Work out the finished part from the listing and answer in its coordinate system (mm). Face numbers are marked on the shaded views. A direction names the side the tool comes from. Round coordinates to 2 decimals unless told otherwise and drop trailing zeros. Order: outer loops, then holes, each group sorted by start corner. A loop starts at its lowest first (then second) coordinate and runs counter-clockwise, first axis right, second up. Notation, with made-up numbers: (-30.5, 29) -> (10.5, 29) arc R11 cw to (10.5, 39) -> close; hole circle Ø3 at (43, -16.75). An arc over 180 degrees is marked (long way). Use a Markdown table: item, result. Add a question column.
Item 1: A cutting plane is placed at C-C, the plane x = 17. Determine the outline of the cut face in (y, z), plus the area to 3 significant figures.
Item 2: A cutting plane is placed at D-D, the plane z = 23.5. Determine the outline of the cut face in (x, y).
Item 3: Find the intervals of material crossed by L1, parallel to Y at x = 62, z = 6.5; L2, parallel to X at y = 72.5, z = 1.5; L3, parallel to Y at x = 41.5, z = 6.75, in increasing order. Write a range as [from, to].
Item 4: For a pull along Y with two mould halves and no side action, classify the marked faces 6, 7, 8 and 9 as +Y half, -Y half, draft (parallel to the pull), parting line (faces both ways), or undercut.
Item 5: A cutting plane is placed at B-B, the plane y = 71. Determine the outline of the cut face in (x, z), plus the area to 3 significant figures.
Item 6: A cutting plane is placed at A-A, the plane z = 9.5. Determine the outline of the cut face in (x, y).
Item 7: A tool of negligible diameter and unlimited length cuts with its end or side. For the marked faces 1, 2, 3, 4 and 5, from which of +Z, -Z, +X, -X, +Y, -Y can it reach the whole face along a straight path? Write none if from no direction.
Item 8: Flat-ended cylindrical pins translate along their axes: P1, Ø5, axis at y = 70, z = 16, coming from the -X side; P2, Ø1, axis at y = 33, z = 9, coming from the -X side; P3, Ø11, axis at x = 56, z = 8, coming from the +Y side. Find the tip coordinate at first contact, or state that the pin passes through.
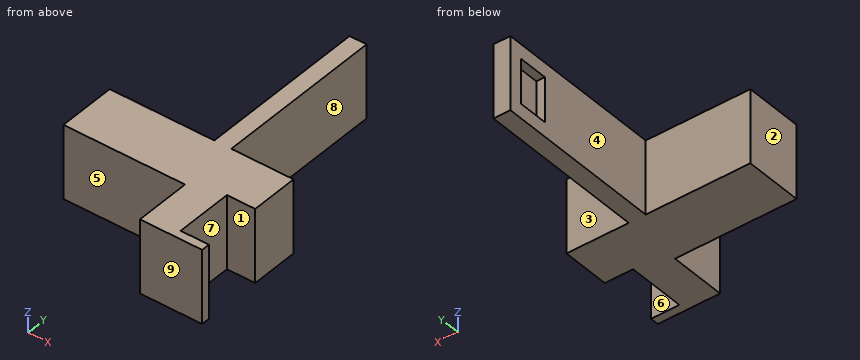
from build123d import *

# Parameters (mm, degrees)
BOSS_EXTRUDE1_DEPTH = 26
SKETCH2_W           = 6
SKETCH2_H           = 26
BOSS_EXTRUDE2_DEPTH = 60
SKETCH3_W           = 15.8
SKETCH3_H           = 10.5
CUT_EXTRUDE1_DEPTH  = 3


with BuildPart() as part:
    # Sketch1 → Boss-Extrude1 (new body)
    with BuildSketch(Plane.XY):
        Polygon((45, 20.52), (65, 20.52), (65, 3.52), (55, 3.52), (55, -17), (65, -17), (65, -20), (43, -20), (43, 0), (0, 0), (0, 20.52), align=None)
    extrude(amount=BOSS_EXTRUDE1_DEPTH)

    # Sketch2 → Boss-Extrude2 (add)
    with BuildSketch(Plane(origin=(0, 20.52, 0), x_dir=(1, 0, 0), z_dir=(0, 1, 0))):
        with Locations((40, -13)):
            Rectangle(SKETCH2_W, SKETCH2_H)
    extrude(amount=BOSS_EXTRUDE2_DEPTH)

    # Sketch3 → Cut-Extrude1 (cut)
    with BuildSketch(Plane.ZY.offset(-37)):
        with Locations((13, 70.52)):
            Rectangle(SKETCH3_W, SKETCH3_H)
    extrude(amount=-CUT_EXTRUDE1_DEPTH, mode=Mode.SUBTRACT)


solid = part.part
Reported:
| question | item | result |
|---|---|---|
| 1 | outline | (0, 0) -> (20.52, 0) -> (20.52, 26) -> (0, 26) -> close |
| 1 | area | 534 mm² |
| 2 | outline | (0, 0) -> (43, 0) -> (43, -20) -> (65, -20) -> (65, -17) -> (55, -17) -> (55, 3.52) -> (65, 3.52) -> (65, 20.52) -> (43, 20.52) -> (43, 80.52) -> (37, 80.52) -> (37, 20.52) -> (0, 20.52) -> close |
| 3 | L1 | [-20, -17], [3.52, 20.52] |
| 3 | L2 | [37, 43] |
| 3 | L3 | [0, 80.52] |
| 4 | face 6 | undercut |
| 4 | face 7 | undercut |
| 4 | face 8 | draft |
| 4 | face 9 | -Y half |
| 5 | outline | (37, 0) -> (43, 0) -> (43, 26) -> (37, 26) -> (37, 20.9) -> (40, 20.9) -> (40, 5.1) -> (37, 5.1) -> close |
| 5 | area | 109 mm² |
| 6 | outline | (0, 0) -> (43, 0) -> (43, -20) -> (65, -20) -> (65, -17) -> (55, -17) -> (55, 3.52) -> (65, 3.52) -> (65, 20.52) -> (43, 20.52) -> (43, 80.52) -> (37, 80.52) -> (37, 75.77) -> (40, 75.77) -> (40, 65.27) -> (37, 65.27) -> (37, 20.52) -> (0, 20.52) -> close |
| 7 | face 1 | +Z, -Z, +X |
| 7 | face 2 | +Z, -Z, -X, +Y, -Y |
| 7 | face 3 | +Z, -Z, +X, +Y |
| 7 | face 4 | +Z, -Z, -X, +Y |
| 7 | face 5 | +Z, -Z, -X, -Y |
| 8 | P1 | x = 40 |
| 8 | P2 | x = 37 |
| 8 | P3 | y = 20.52 |
